Source: CAD feature listing. Evaluate the final solid. Frame: model axes, mm. Face numbers are marked on the shaded views. A direction names the side the tool comes from. Coordinates: 2 decimals unless noted, no trailing zeros. Write each loop counter-clockwise with the first axis right and the second up, starting at its lowest first coordinate (ties: lowest second). Pieces come first, ordered by that corner, then holes. Notation, with made-up numbers: (69, 23.25) -> (103, 23.25) arc R10 ccw to (103, 36.25) -> close; hole circle Ø6 at (66.25, 40). An arc over 180 degrees is marked (long way). Write item = value, one per line.
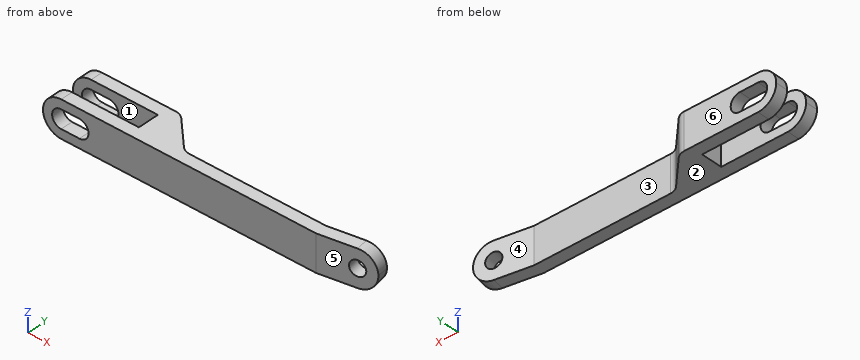
from build123d import *

# Parameters (mm, degrees)
F1_DEPTH = 6
F3_DEPTH = 25
F4_R     = 2.99999
F5_R     = 1.25
F6_DEPTH = 25
F7_R     = 2.99999


# Not quite as in the source:
# - a fillet or chamfer is up to 0.001 mm smaller than in the source, because OpenCascade refuses the exact size


with BuildPart() as f1:
    # F0 (on Top) → F1 (new body)
    with BuildSketch(Plane.XY):
        with BuildLine():
            Line((-22.5, -1), (22.5, -1))
            Line((22.5, -1), (31.3632697771, 0.562833599))
            Line((31.3632697771, 0.562833599), (31.0159734218, 2.532449105))
            Line((31.0159734218, 2.532449105), (22.3250226729, 1))
            Line((22.3250226729, 1), (-0.1715728753, 1))
            ThreePointArc((-0.1715728753, 1), (-0.93693974, 1.152240935), (-1.5857864376, 1.5857864376))
            Line((-1.5857864376, 1.5857864376), (-5.9142135624, 5.9142135624))
            ThreePointArc((-5.9142135624, 5.9142135624), (-6.56306026, 6.347759065), (-7.3284271247, 6.5))
            Line((-7.3284271247, 6.5), (-22.5, 6.5))
            Line((-22.5, 6.5), (-22.5, 4.5))
            Line((-22.5, 4.5), (-8.5, 4.5))
            Line((-8.5, 4.5), (-8.5, 1))
            Line((-8.5, 1), (-22.5, 1))
            Line((-22.5, 1), (-22.5, -1))
        make_face()
    extrude(amount=F1_DEPTH)

    # F2 (on face) → F3 (cut)
    with BuildSketch(Plane.XZ.offset(1)):
        with BuildLine():
            Line((-16.5, 4.5), (-19.5, 4.5))
            ThreePointArc((-19.5, 4.5), (-21, 2.999998177), (-19.499996354, 1.5))
            Line((-19.499996354, 1.5), (-16.5046735253, 1.5000072806))
            ThreePointArc((-16.5046735253, 1.5000072806), (-15.0000018202, 2.9976632345), (-16.5, 4.5))
        make_face()
    extrude(amount=-F3_DEPTH, mode=Mode.SUBTRACT)

    # F4 (radius 3 in the source; OpenCascade refuses exactly that, so slightly less here)
    f4_edges = [f1.edges().sort_by_distance(p)[0] for p in [
        (-22.5, 5.5, 6),
        (-22.5, 0, 6),
        (-22.5, 5.5, 0),
        (-22.5, 0, 0),
    ]]
    fillet(f4_edges, radius=F4_R)

    # F5 (on face) → F6 (cut)
    with BuildSketch(Plane(origin=(0.8494680878, -4.8175729228, 0), x_dir=(0.984807753, 0.1736481777, 0), z_dir=(0.1736481777, -0.984807753, 0))):
        with Locations((27.9845262651, 3)):
            Circle(F5_R)
    extrude(amount=-F6_DEPTH, mode=Mode.SUBTRACT)

    # F7 (radius 3 in the source; OpenCascade refuses exactly that, so slightly less here)
    f7_edges = [f1.edges().sort_by_distance(p)[0] for p in [
        (31.189622, 1.547641, 6),
        (31.189622, 1.547641, 0),
    ]]
    fillet(f7_edges, radius=F7_R)


solid = f1.part
1) Reachability of the marked faces 1 and 2 from +Z, -Z, +X, -X, +Y, -Y: full face, straight path, thin tool, end or side. Return the list, or none.
Answer block:
face_1 = +Z, -Z, -X
face_2 = -Z, +X, -X, +Y, -Y
2) Material intervals for probe 1 along Y at (x, z) = (21, 2); probe 2 along X at (y, z) = (2, 3); probe 3 along X at (y, z) = (5.5, 1), sorted ascending. Write a range as [from, to].
Answer block:
probe_1 = [-1, 1]
probe_2 = [-8.5, -2], [29.33, 31.11]
probe_3 = [-21.74, -5.5]
3) Pull-direction query (X, two-part tool) for the marked faces 3, 4, 5 and 6; classes: +X half, -X half, draft (parallel to the pull), parting line (faces both ways), or undercut.
Answer block:
face_3 = undercut
face_4 = undercut
face_5 = +X half
face_6 = draft
4) Cut plane A-A, the plane z = 2.5. Output: boundary loops of the cut face in (x, y), and give its area (3 significant figures).
Answer block:
outline = (-22.46, -1) -> (-20.91, -1) -> (-20.91, 1) -> (-22.46, 1) -> close; (-22.46, 4.5) -> (-20.91, 4.5) -> (-20.91, 6.5) -> (-22.46, 6.5) -> close; (-15.09, -1) -> (22.5, -1) -> (27.28, -0.16) -> (26.93, 1.81) -> (22.33, 1) -> (-0.17, 1) arc R2 cw to (-1.59, 1.59) -> (-5.91, 5.91) arc R2 ccw to (-7.33, 6.5) -> (-15.09, 6.5) -> (-15.09, 4.5) -> (-8.5, 4.5) -> (-8.5, 1) -> (-15.09, 1) -> close; (29.19, 2.21) -> (29.54, 0.24) -> (31.32, 0.56) -> (30.97, 2.53) -> close
area = 134 mm2
5) Cut plane D-D, the plane z = 0.5. Output: boundary loops of the cut face in (x, y), and give its area (3 significant figures).
Answer block:
outline = (-21.16, -1) -> (22.5, -1) -> (30.04, 0.33) -> (29.69, 2.3) -> (22.33, 1) -> (-0.17, 1) arc R2 cw to (-1.59, 1.59) -> (-5.91, 5.91) arc R2 ccw to (-7.33, 6.5) -> (-21.16, 6.5) -> (-21.16, 4.5) -> (-8.5, 4.5) -> (-8.5, 1) -> (-21.16, 1) -> close
area = 154 mm2
6) Cut plane B-B, the plane x = 19.5. Output: boundary loops of the cut face in (y, z), and give its area (3 significant figures).
Answer block:
outline = (-1, 0) -> (1, 0) -> (1, 6) -> (-1, 6) -> close
area = 12.0 mm2
7) First-contact query: pin 1 Ø1.8 at (x, z) = (12, 3.5) entering from +Y. Flat tip, straight axial feed; report the tip coordinate or a pass-through.
Answer block:
pin_1 = 1
8) Cut plane C-C, the plane y = 3.75. Output: boundary loops of the cut face in (x, z), and give its area (3 significant figures).
Answer block:
outline = (-8.5, 0) -> (-3.75, 0) -> (-3.75, 6) -> (-8.5, 6) -> close
area = 28.5 mm2
